```python
from build123d import *

# Parameters (mm, degrees)
BOSS_EXTRUDE1_DEPTH = 10
CUT_EXTRUDE2_DEPTH  = 10
BOSS_EXTRUDE2_DEPTH = 10
SKETCH7_R           = 15
CUT_EXTRUDE3_DEPTH  = 17
SKETCH8_R           = 15
BOSS_EXTRUDE4_DEPTH = 2
SKETCH10_R          = 4
BOSS_EXTRUDE5_DEPTH = 7
FILLET1_R           = 10
CUT_EXTRUDE4_DEPTH  = 10
FILLET2_R           = 10
SKETCH12_W          = 25
SKETCH12_H          = 10
CUT_EXTRUDE5_DEPTH  = 5
SKETCH13_R          = 1.505
CUT_EXTRUDE6_DEPTH  = 15
BOSS_EXTRUDE6_DEPTH = 10


with BuildPart() as part:
    # Sketch2 → Boss-Extrude1 (new body)
    with BuildSketch(Plane.XY):
        with BuildLine():
            Line((0, 0), (70, 0))
            ThreePointArc((70, 0), (80.047115298, 146.372811683), (110, 290))
            Line((110, 290), (50, 290))
            ThreePointArc((50, 290), (12.591539765, 147.139389696), (0, 0))
        make_face()
    extrude(amount=BOSS_EXTRUDE1_DEPTH)

    # Sketch5 → Cut-Extrude2 (cut)
    with BuildSketch(Plane.XY.offset(10)):
        Polygon((-13.167731947, 80), (152.833861951, 80), (152.833861951, 337.050867126), (18.976855574, 332.054655913), align=None)
    extrude(amount=-CUT_EXTRUDE2_DEPTH, mode=Mode.SUBTRACT)

    # Sketch6 → Boss-Extrude2 (add)
    with BuildSketch(Plane.XY.offset(10)):
        Polygon((72.991341013, 80), (3.703067383, 80), (44.276364493, 147.051943441), align=None)
    extrude(amount=-BOSS_EXTRUDE2_DEPTH)

    # Sketch7 → Cut-Extrude3 (cut)
    with BuildSketch(Plane(origin=(0, 0, 0), x_dir=(-1, 0, 0), z_dir=(0, 0, -1))):
        with Locations((-44.276364493, 147.051943441)):
            Circle(SKETCH7_R)
    extrude(amount=-CUT_EXTRUDE3_DEPTH, mode=Mode.SUBTRACT)

    # Fillet1
    fillet1_edges = [part.edges().sort_by_distance(p)[0] for p in [
        (3.703067383, 80, 5),
        (72.991341013, 80, 5),
    ]]
    fillet(fillet1_edges, radius=FILLET1_R)

    # Sketch11 → Cut-Extrude4 (cut)
    with BuildSketch(Plane.XY.offset(10)):
        Polygon((13.865882816, 96.79519719), (9.525195507, -12.111976015), (-19.82973313, -10.941983603), (-15.53567793, 96.79519719), align=None)
    extrude(amount=-CUT_EXTRUDE4_DEPTH, mode=Mode.SUBTRACT)

    # Fillet2
    fillet2_edges = [part.edges().sort_by_distance(p)[0] for p in [
        (13.865882816, 96.79519719, 5),
    ]]
    fillet(fillet2_edges, radius=FILLET2_R)

    # Sketch12 → Cut-Extrude5 (cut)
    with BuildSketch(Plane(origin=(0, 0, 0), x_dir=(-1, 0, 0), z_dir=(0, 0, -1))):
        with Locations((-37.5, 5)):
            Rectangle(SKETCH12_W, SKETCH12_H)
    extrude(amount=-CUT_EXTRUDE5_DEPTH, mode=Mode.SUBTRACT)

    # Sketch13 → Cut-Extrude6 (cut)
    with BuildSketch(Plane(origin=(0, 0, 5), x_dir=(-1, 0, 0), z_dir=(0, 0, -1))):
        with Locations((-45, 5)):
            Circle(SKETCH13_R)
        with Locations((-37.5, 5)):
            Circle(SKETCH13_R)
        with Locations((-30, 5)):
            Circle(SKETCH13_R)
    extrude(amount=-CUT_EXTRUDE6_DEPTH, mode=Mode.SUBTRACT)



with BuildPart() as body_2:
    # Sketch8 → Boss-Extrude4 (new body)
    with BuildSketch(Plane(origin=(0, 0, 0), x_dir=(-1, 0, 0), z_dir=(0, 0, -1))):
        with Locations((-44.276364493, 147.051943441)):
            Circle(SKETCH8_R)
    extrude(amount=-BOSS_EXTRUDE4_DEPTH)

    # Sketch10 → Boss-Extrude5 (add)
    with BuildSketch(Plane.XY.offset(2)):
        with Locations((44.276364493, 147.051943441)):
            Circle(SKETCH10_R)
    extrude(amount=BOSS_EXTRUDE5_DEPTH)


with BuildPart() as part_1:
    add(part.part)

    add(body_2.part)  # Boss-Extrude6 merges body 2
    # Sketch14 → Boss-Extrude6 (add)
    with BuildSketch(Plane(origin=(0, 0, 0), x_dir=(-1, 0, 0), z_dir=(0, 0, -1))):
        with BuildLine():
            Line((-53.147136244, 126.337927349), (-55.598718025, 137.213025284))
            ThreePointArc((-55.598718025, 137.213025284), (-56.912855269, 139.008842213), (-57.946701254, 140.97939483))
            Line((-57.946701254, 140.97939483), (-54.372927134, 123.47560004))
            Line((-54.372927134, 123.47560004), (-53.147136244, 126.337927349))
        make_face()
        with BuildLine():
            ThreePointArc((-31.612557589, 139.012789587), (-32.24957103, 138.087779286), (-32.954010961, 137.213025284))
            Line((-32.954010961, 137.213025284), (-31.742262033, 126.337927349))
            Line((-31.742262033, 126.337927349), (-29.852240994, 123.214454699))
            Line((-29.852240994, 123.214454699), (-31.612557589, 139.012789587))
        make_face()
    extrude(amount=-BOSS_EXTRUDE6_DEPTH)


solid = part_1.part
```
The listing builds one solid part. Answer for the finished solid, in the listing's coordinates (mm). A direction names the side the tool comes from. Coordinates: 2 decimals unless noted, no trailing zeros. Loops run counter-clockwise (first coordinate to the right, second up) from the corner with the lowest first, then second, coordinate; pieces in that order, holes last. Notation, with made-up numbers: M 64.5,46 L 74.5,46 A25 ccw 74.5,65 Z; hole C 65.25,51.5 d10. An arc over 180 degrees is marked long. Answer as a JSON object with one key per item and string values. Group by question number.
Item 1: Consider L1, parallel to Y at x = 45, z = 8.8 (3 decimals); L2, parallel to Y at x = 37.5, z = 7.7 (3 decimals); L3, parallel to X at y = 49, z = 6.5. Determine where each line is inside the solid, lowest interval first.
Item 2: Section B-B (x = 45) is taken. Write down the section's boundary in (y, z) (3 decimals), and give its area (3 significant figures).
Item 3: Section D-D (y = 86.5) is taken. Write down the section's boundary in (x, z).
Item 4: Which of the six approach directions +Z, -Z, +X, -X, +Y, -Y give full straight-line access (tool end or side, diameter ignored) to faces 5 (the face through (41, 144, 2)), 6 (the face through (56.185, 132.35, 4.93)), 7 (the face through (25, 5, 2))?
Item 5: Determine the mould class of faces 1 (the face through (72.707, 79.924, 4.93)), 2 (the face through (46.427, 150.425, 5.451)), 3 (the face through (32.357, 131.852, 4.93)), 4 (the face through (53.15, 134.96, 0.99)) for opening direction X: +X half, -X half, draft (parallel to the pull), parting line (faces both ways), or undercut.
Item 6: Section C-C (y = 5) is taken. Write down the section's boundary in (x, z) (3 decimals), and give its area (3 significant figures).
Item 7: Section A-A (z = 6.5) is taken. Write down the section's boundary in (x, y) (3 decimals), and give its area (3 significant figures).
Item 8: Each of these flat-tipped pins is pushed along its axis until it touches: P1, Ø2.5, axis at x = 30, y = 5, coming from the +Z side; P2, Ø1.5, axis at x = 31.5, z = 2, coming from the -Y side; P3, Ø5, axis at x = 45, y = 5, coming from the -Z side; P4, Ø1, axis at y = 113.5, z = 7, coming from the +X side. Where does it stop, or does it pass through?
Solved:
{
 "1": {"L1": "y = 0 to 3.495, 6.505 to 132.069, 143.118 to 150.986", "L2": "y = 0 to 3.495, 6.505 to 133.67", "L3": "x = 11.96 to 71.12"},
 "2": {"outline": "M 0,5 L 3.495,5 L 3.495,10 L 0,10 Z; M 6.505,5 L 10,5 L 10,0 L 162.034,0 L 162.034,2 L 150.986,2 L 150.986,9 L 143.118,9 L 143.118,2 L 132.069,2 L 132.069,10 L 6.505,10 Z", "area": "1,370 mm2"},
 "3": {"outline": "M 13.46,0 L 70.21,0 L 70.21,10 L 13.46,10 Z"},
 "4": {"face 5": "+Z", "face 6": "+Z, -Z, +X", "face 7": "-Z, -Y"},
 "5": {"face 1": "+X half", "face 2": "parting line", "face 3": "undercut", "face 4": "undercut"},
 "6": {"outline": "M 10.207,0 L 25,0 L 25,5 L 28.495,5 L 28.495,10 L 10.207,10 Z; M 31.505,5 L 35.995,5 L 35.995,10 L 31.505,10 Z; M 39.005,5 L 43.495,5 L 43.495,10 L 39.005,10 Z; M 46.505,5 L 50,5 L 50,0 L 70.012,0 L 70.012,10 L 46.505,10 Z", "area": "428 mm2"},
 "7": {"outline": "M 10.008,0 L 70,0 A1071.25 cw 72.813,77.58 A10 ccw 72.032,82.241 L 54.373,123.476 L 57.947,140.979 A14.992 cw 55.599,137.213 L 53.147,126.338 L 50.181,133.263 A15 cw 36.511,134.219 L 31.742,126.338 L 32.954,137.213 A15 cw 31.613,139.013 L 29.852,123.214 L 15.2,99 A10 ccw 13.763,94.221 Z; C 44.276,147.052 d8; hole C 30,5 d3.01; hole C 37.5,5 d3.01; hole C 45,5 d3.01", "area": "6,960 mm2"},
 "8": {"P1": "passes through", "P2": "stops at y = 10", "P3": "stops at z = 5", "P4": "stops at x = 58.86"}
}
